The drawing under review shows one solid part. Ordinate dimensions are in mm from its lowest x, y, z. A direction names the side the tool comes from. Round coordinates to 2 decimals unless told otherwise and drop trailing zeros. Write each loop counter-clockwise with the first axis right and the second up, starting at its lowest first coordinate (ties: lowest second). Pieces come first, ordered by that corner, then holes. Notation, with made-up numbers: (26.25, 59) -> (38.25, 59) arc R9 cw to (38.25, 75) -> close; hole circle Ø1 at (77, -25). An arc over 180 degrees is marked (long way). Write item = value, one per line. Start each with the question number.
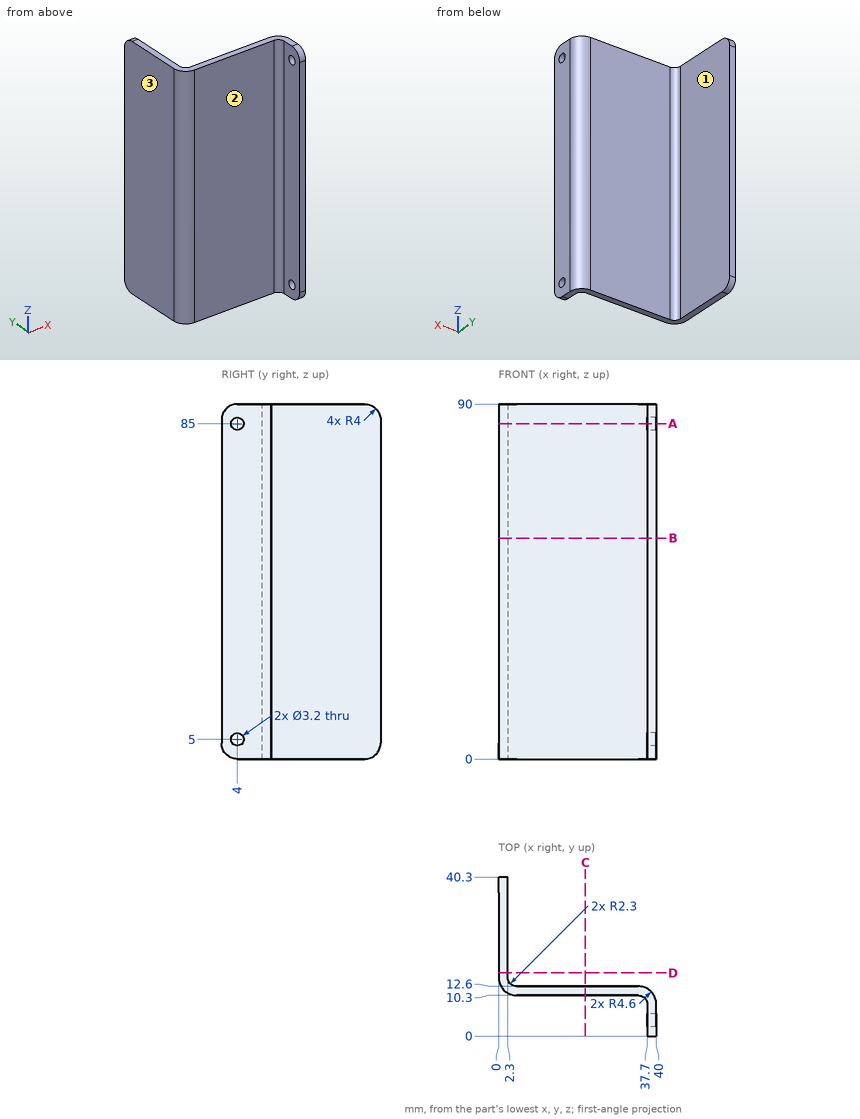
1. Wall thickness on L1, parallel to Y at x = 12.5, z = 10; L2, parallel to X at y = 8, z = 59; L3, parallel to X at y = 30.5, z = 31: over which ranges is each line inside the solid? List them lowest first. Write a range as from..to.
2. Machinability: for the marked faces 1, 2 and 3, which of the approach directions +Z, -Z, +X, -X, +Y, -Y give a long, thin tool a straight path to every point of the face, cutting with its end or side? Answer none if there is none.
3. Clearance check with flat-ended pins moving along their axes: pin 1 Ø1 at (x, z) = (13, 12) entering from +Y; pin 2 Ø7.5 at (y, z) = (24, 47) entering from +X; pin 3 Ø1.9 at (y, z) = (4, 85) entering from +X; pin 4 Ø6.5 at (y, z) = (4, 37) entering from -X. State where each tip first meets the part, or that it passes through.
4. Consider section C-C, the plane x = 22. Give the boundary of the cut face in (y, z), then the cut area to 3 significant figures.
5. Consider section D-D, the plane y = 16. Give the boundary of the cut face in (x, z).
6. Consider section A-A, the plane z = 85. Give the boundary of the cut face in (x, y), then the cut area to 3 significant figures.
7. Consider section B-B, the plane z = 56. Give the boundary of the cut face in (x, y), then the cut area to 3 significant figures.
Outcome:
q1.L1 = 10.3..12.6
q1.L2 = 37.7..40
q1.L3 = 0..2.3
q2.face_1 = +Z, -Z, +X, +Y
q2.face_2 = +Z, -Z, -X, -Y
q2.face_3 = +Z, -Z, -X, +Y, -Y
q3.pin_1 = 12.6
q3.pin_2 = 2.3
q3.pin_3 = through
q3.pin_4 = 37.7
q4.outline = (10.3, 0) -> (12.6, 0) -> (12.6, 90) -> (10.3, 90) -> close
q4.area = 207 mm2
q5.outline = (0, 0) -> (2.3, 0) -> (2.3, 90) -> (0, 90) -> close
q6.outline = (0, 14.9) arc R4.6 ccw to (4.6, 10.3) -> (35.4, 10.3) arc R2.3 cw to (37.7, 8) -> (37.7, 5.6) -> (40, 5.6) -> (40, 8) arc R4.6 ccw to (35.4, 12.6) -> (4.6, 12.6) arc R2.3 cw to (2.3, 14.9) -> (2.3, 40.3) -> (0, 40.3) -> close; (37.7, 0) -> (40, 0) -> (40, 2.4) -> (37.7, 2.4) -> close
q6.area = 165 mm2
q7.outline = (0, 14.9) arc R4.6 ccw to (4.6, 10.3) -> (35.4, 10.3) arc R2.3 cw to (37.7, 8) -> (37.7, 0) -> (40, 0) -> (40, 8) arc R4.6 ccw to (35.4, 12.6) -> (4.6, 12.6) arc R2.3 cw to (2.3, 14.9) -> (2.3, 40.3) -> (0, 40.3) -> close
q7.area = 173 mm2
